Build history of the part. All positions in model axes, mm. A direction names the side the tool comes from. Give positions to 0.01 mm unless a question says otherwise; leave off trailing zeros. Order: outer loops, then holes, each group sorted by start corner. A loop starts at its lowest first (then second) coordinate and runs counter-clockwise, first axis right, second up. Notation, with made-up numbers: (49, 30) - (82, 30) arc R12 ccw to (82, 44) - close; hole circle Ø11 at (12.25, -16.75). An arc over 180 degrees is marked (long way). Use a Markdown table: item, result.
Autodesk Inventor part; units mm, degrees
ref_plane "YZ Plane" through (0, 0, 0) normal (1, 0, 0) x (0, 1, 0)
ref_plane "XZ Plane" through (0, 0, 0) normal (0, 1, 0) x (-1, 0, 0)
ref_plane "XY Plane" through (0, 0, 0) normal (0, 0, 1) x (1, 0, 0)
sketch "Sketch1" plane through (0, 0, 0) normal (0, 0, 1) x (1, 0, 0)
  line L0 (-79.2915, 39.2514) -> (-13.7915, 39.2514)
  line L1 (-13.7915, 39.2514) -> (-13.7915, 1.2514)
  line L2 (-13.7915, 1.2514) -> (-79.2915, 1.2514)
  line L3 (-79.2915, 1.2514) -> (-79.2915, 39.2514)
  point P0 (0, 0)
extrude "Extrusion1" add sketch "Sketch1" along normal blind 1.5
sketch "Sketch2" plane through (0, 0, 1.5) normal (0, 0, 1) x (1, 0, 0)
  line L0 (-13.7915, 39.2514) -> (-13.7915, 1.2514)
  line L1 (-79.2915, 39.2514) -> (-13.7915, 39.2514)
  line L2 (-79.2915, 1.2514) -> (-79.2915, 39.2514)
  line L3 (-13.7915, 1.2514) -> (-79.2915, 1.2514)
  line L4 (-79.2915, 37.2514) -> (-15.7915, 37.2514)
  line L5 (-15.7915, 37.2514) -> (-15.7915, 3.2514)
  line L6 (-15.7915, 3.2514) -> (-79.2915, 3.2514)
  point P0 (0, 0)
  dimension "d2" = 2
  dimension "d3" = 2
  dimension "d4" = 2
extrude "Extrusion2" add sketch "Sketch2" along normal blind 14.5 contours L0 L3 L2 L6 L5 L4 L1
sketch "Sketch3" plane through (-13.7915, 1.2514, 0) normal (1, 0, 0) x (0, 0, -1)
  line L0 (0, 0) -> (-16, 0)
  line L1 (0, 38) -> (0, 0)
  line L2 (0, 38) -> (-16, 38)
  line L3 (-16, 38) -> (-16, 0)
  arc A0 (-13, 24.3) -> (-13, 30.7) centre (-13, 27.5) ccw
  line L4 (-13, 30.7) -> (-16, 30.7)
  line L5 (-13, 24.3) -> (-16, 24.3)
  arc A1 (-13, 7.3) -> (-13, 13.7) centre (-13, 10.5) ccw
  line L6 (-13, 7.3) -> (-16, 7.3)
  line L7 (-13, 13.7) -> (-16, 13.7)
  point P0 (0, -1.2514)
  dimension "d7" = 13
  dimension "d8" = 10.5
  dimension "d9" = 3.2
  dimension "d10" = 13
  dimension "d11" = 10.5
extrude "Extrusion3" cut sketch "Sketch3" against normal blind 13 contours L3 L7 A1 L6 | L4 A0 L5 L3
sketch "Sketch4" plane through (0, 0, 0) normal (0, 0, -1) x (-1, 0, 0)
  line L0 (21.3312, 42.5198) -> (19.2419, 38.901)
  arc A0 (21.3312, 42.5198) -> (21.3312, 44.5198) centre (19.5992, 43.5198) ccw
  line L1 (19.8192, 47.1386) -> (21.3312, 44.5198)
  arc A1 (19.8192, 47.1386) -> (18.0872, 48.1386) centre (18.0872, 46.1386) ccw
  line L2 (15.0633, 48.1386) -> (18.0872, 48.1386)
  arc A2 (15.0633, 48.1386) -> (13.3312, 47.1386) centre (15.0633, 46.1386) ccw
  line L3 (11.8192, 44.5198) -> (13.3312, 47.1386)
  arc A3 (11.8192, 44.5198) -> (11.8192, 42.5198) centre (13.5513, 43.5198) ccw
  line L4 (12.8585, 40.7198) -> (11.8192, 42.5198)
  circle A4 centre (16.5752, 43.5198) radius 1.65
  line L5 (12.8585, 40.7198) -> (13.7938, 39.0998)
  line L6 (13.7938, 39.0998) -> (19.3567, 39.0998)
  point P0 (0, 0)
  point P1 (16.0419, 38.7198)
extrude "Extrusion4" add sketch "Sketch4" against normal blind 16
sketch "Sketch5" plane through (-79.2915, 1.2514, 0) normal (-1, 0, 0) x (0, 0, 1)
  line L0 (1.5, 2) -> (1.5, 36)
  line L1 (0, 38) -> (16, 38)
  line L2 (0, 0) -> (0, 38)
  line L3 (0, 0) -> (16, 0)
  line L4 (1.5, 36) -> (1.5, 38)
  line L5 (1.5, 2) -> (1.5, 0)
  point P0 (0, -1.2514)
extrude "Extrusion5" add sketch "Sketch5" along normal blind 8
sketch "Sketch6" plane through (0, 0, 1.5) normal (0, 0, 1) x (1, 0, 0)
  line L0 (-15.7915, 37.2514) -> (-79.2915, 37.2514)
  line L1 (-79.2915, 3.2514) -> (-15.7915, 3.2514)
  line L2 (-15.7915, 3.2514) -> (-15.7915, 37.2514)
  line L3 (-69.2915, 37.2514) -> (-66.2915, 37.2514)
  line L4 (-66.2915, 37.2514) -> (-66.2915, 3.2514)
  line L5 (-66.2915, 3.2514) -> (-69.2915, 3.2514)
  line L6 (-69.2915, 3.2514) -> (-69.2915, 37.2514)
  line L7 (-40.7915, 37.2514) -> (-37.7915, 37.2514)
  line L8 (-37.7915, 37.2514) -> (-37.7915, 3.2514)
  line L9 (-37.7915, 3.2514) -> (-40.7915, 3.2514)
  line L10 (-40.7915, 3.2514) -> (-40.7915, 37.2514)
  point P0 (0, 0)
  dimension "d18" = 3
  dimension "d19" = 3
  dimension "d20" = 22
  dimension "d21" = 10
extrude "Extrusion6" add sketch "Sketch6" along normal blind 5.2 contours L8 L1 L10 L0 | L4 L1 L6 L0
sketch "Sketch7" plane through (0, 0, 0) normal (0, 0, -1) x (-1, 0, 0)
  line L0 (87.2915, 39.2514) -> (19.4442, 39.2514)
  line L1 (18.0872, 35.2514) -> (20.0872, 35.2514)
  line L2 (20.0872, 35.2514) -> (20.0872, 5.2514)
  line L3 (20.0872, 5.2514) -> (18.0872, 5.2514)
  line L4 (18.0872, 5.2514) -> (18.0872, 35.2514)
  circle A0 centre (19.0872, 35.2514) radius 1
  circle A1 centre (19.0872, 5.2514) radius 1
  point P0 (0, 0)
  dimension "d24" = 2
  dimension "d25" = 30
  dimension "d26" = 4
  dimension "d32" = 2
  dimension "d33" = 2
extrude "Extrusion7" cut sketch "Sketch7" against normal blind 2
pattern_linear "Rectangular Pattern1" count 5 spacing 4 along (-1, 0, 0) of "Extrusion7"
sketch "Sketch8" plane through (0, 0, 0) normal (0, 0, -1) x (-1, 0, 0)
  line L0 (13.7915, 1.2514) -> (87.2915, 1.2514)
  line L1 (87.2915, 1.2514) -> (87.2915, 39.2514)
  line L2 (42.2915, 32.2514) -> (44.2915, 32.2514)
  line L3 (44.2915, 32.2514) -> (44.2915, 8.2514)
  line L4 (44.2915, 8.2514) -> (42.2915, 8.2514)
  line L5 (42.2915, 8.2514) -> (42.2915, 32.2514)
  circle A0 centre (43.2915, 32.2514) radius 1
  circle A1 centre (43.2915, 8.2514) radius 1
  point P0 (0, 0)
  dimension "d34" = 2
  dimension "d35" = 24
  dimension "d36" = 43
  dimension "d37" = 7
extrude "Extrusion8" cut sketch "Sketch8" against normal blind 2
pattern_linear "Rectangular Pattern2" count 2 spacing 4 along (-1, 0, 0) of "Extrusion8"
sketch "Sketch9" plane through (0, 0, 0) normal (0, 0, -1) x (-1, 0, 0)
  line L0 (87.2915, 39.2514) -> (19.4442, 39.2514)
  line L1 (55.3139, 35.2514) -> (57.3139, 35.2514)
  line L2 (57.3139, 35.2514) -> (57.3139, 5.2514)
  line L3 (57.3139, 5.2514) -> (55.3139, 5.2514)
  line L4 (55.3139, 5.2514) -> (55.3139, 35.2514)
  circle A0 centre (56.3139, 35.2514) radius 1
  circle A1 centre (56.3139, 5.2514) radius 1
  point P0 (0, 0)
  dimension "d43" = 30
  dimension "d44" = 4
extrude "Extrusion9" cut sketch "Sketch9" against normal blind 2
pattern_linear "Rectangular Pattern3" count 3 spacing 4 along (-1, 0, 0) of "Extrusion9"
sketch "Sketch11" plane through (0, 0, 0) normal (0, 0, -1) x (-1, 0, 0)
  line L0 (87.2915, 1.2514) -> (87.2915, 39.2514)
  line L1 (87.2915, 39.2514) -> (19.4442, 39.2514)
  circle A0 centre (84.7915, 32.3514) radius 1.5
  circle A1 centre (84.7915, 8.1514) radius 1.5
  point P0 (0, 0)
  dimension "d50" = 2.5
  dimension "d51" = 2.5
  dimension "d52" = 24.2
  dimension "d53" = 6.9
extrude "Extrusion10" cut sketch "Sketch11" against normal blind 10
chamfer "Chamfer1" distance 0.5 angle 45 13 edges at (-50.5415, 1.2514, 0) (-13.7915, 20.1776, 0) (-13.7915, 1.2514, 8) (-53.3678, 39.2514, 0) (-20.3877, 40.8856, 0) (-21.5992, 43.5198, 0) (-20.5752, 45.8292, 0) (-19.0872, 47.8707, 0) (-16.5752, 48.1386, 0) (-14.0633, 47.8707, 0) (-12.5752, 45.8292, 0) (-11.5513, 43.5198, 0) (-12.8054, 40.8118, 0)
sketch "Sketch12" plane through (0, 0, 0) normal (0, 0, -1) x (-1, 0, 0)
  line L0 (87.2915, 1.7514) -> (87.2915, 38.7514)
  circle A0 centre (84.7915, 32.3514) radius 1.5
  circle A1 centre (84.7915, 8.1514) radius 1.5
  line L1 (87.2915, 39.2514) -> (79.2915, 39.2514)
  line L2 (79.2915, 39.2514) -> (79.2915, 1.2514)
  line L3 (79.2915, 1.2514) -> (87.2915, 1.2514)
  line L4 (87.2915, 1.2514) -> (87.2915, 39.2514)
  line L5 (14.2915, 1.2514) -> (87.2915, 1.2514)
  point P0 (0, 0)
  dimension "d59" = 38
  dimension "d60" = 8
  dimension "d61" = 0
  dimension "d64" = 0
extrude "Extrusion11" add sketch "Sketch12" against normal blind 1
sketch "Sketch13" plane through (0, 0, 0) normal (0, 0, -1) x (-1, 0, 0)
  circle A0 centre (16.5752, 43.5198) radius 1.65
  circle A1 centre (16.5752, 43.5198) radius 3.5
  point P0 (0, 0)
extrude "Extrusion12" cut sketch "Sketch13" against normal blind 3
properties part number "case add on sdr botom"
1) Two-plate mould, pull along Y, no slides. Class faces 1 (the flat face through (-35, 38, 16)), 2 (the cylindrical face through (-19.1, 47.863, 8.142)), 3 (the flat face through (-66.292, 20, 4)): +Y half, -Y half, draft (parallel to the pull), parting line (faces both ways), or undercut.
Computed:
| item | result |
|---|---|
| face 1 | draft |
| face 2 | +Y half |
| face 3 | undercut |
2) Tool access for faces 4 (the flat face through (-29, 20, 1.5)), 5 (the flat face through (-79.292, 38, 9)), 6 (the flat face through (-39, 20, 6.7)), 7 (the cylindrical face through (-27.07, 4.25, 0.74)): list every direction of +Z, -Z, +X, -X, +Y, -Y with a clear straight run to the whole face (end or side of a thin tool).
Computed:
| item | result |
|---|---|
| face 4 | +Z |
| face 5 | +Z, -X, +Y, -Y |
| face 6 | +Z, -X |
| face 7 | +Z, -Z |
3) Wall check: line 1 (X direction, y = 32.5, z = 1.75); line 2 (Y direction, x = -60.5, z = 6.25); line 3 (X direction, y = 36, z = 12.75). Give the ranges that are in metal, low to high. Write a range as from..to.
Computed:
| item | result |
|---|---|
| line 1 | x = -69.29..-66.29, -40.79..-37.79, -15.79..-13.79 |
| line 2 | y = 1.25..3.25, 37.25..39.25 |
| line 3 | x = -15.79..-13.79 |
4) Slice it at D-D (y = 30). State how many separate pieces and enclosed holes the cut face has, and give its area (3 significant figures).
Computed:
| item | result |
|---|---|
| separate pieces | 11 |
| enclosed holes | 0 |
| area | 128 mm² |
5) Slice it at C-C (z = 4.75). Write the cut outline in (x, y).
Computed:
| item | result |
|---|---|
| outline | (-79.29, 1.25) - (-14.29, 1.25) - (-13.79, 1.75) - (-13.79, 39.1) - (-12.86, 40.72) - (-11.82, 42.52) arc R2 ccw to (-11.82, 44.52) - (-13.33, 47.14) arc R2 ccw to (-15.06, 48.14) - (-18.09, 48.14) arc R2 ccw to (-19.82, 47.14) - (-21.33, 44.52) arc R2 ccw to (-21.33, 42.52) - (-19.44, 39.25) - (-79.29, 39.25) - (-79.29, 37.25) - (-69.29, 37.25) - (-69.29, 3.25) - (-79.29, 3.25) - close; hole (-66.29, 3.25) - (-40.79, 3.25) - (-40.79, 37.25) - (-66.29, 37.25) - close; hole (-37.79, 3.25) - (-15.79, 3.25) - (-15.79, 37.25) - (-37.79, 37.25) - close; hole circle Ø3.3 at (-16.58, 43.52) |
6) Slice it at B-B (y = 38). Write the cut outline in (x, z).
Computed:
| item | result |
|---|---|
| outline | (-87.29, 0) - (-14.29, 0) - (-13.79, 0.5) - (-13.79, 16) - (-79.29, 16) - (-79.29, 1.5) - (-87.29, 1.5) - close |
7) Pin check, flat tips, straight feed: P1, Ø3.5, axis at x = -67.5, y = 17, coming from the +Z side; P2, Ø4, axis at x = -84.79, y = 8.15, coming from the +Z side; P3, Ø0.6, axis at y = 1.5, z = 0.5, coming from the +X side. Stop position of each tip, or through.
Computed:
| item | result |
|---|---|
| P1 | stops at z = 6.7 |
| P2 | stops at z = 1.5 |
| P3 | stops at x = -13.79 |
8) Slice it at A-A (z = 15). Write the cut outline in (x, y).
Computed:
| item | result |
|---|---|
| outline | (-79.29, 1.25) - (-14.29, 1.25) - (-13.79, 1.75) - (-13.79, 8.55) - (-15.79, 8.55) - (-15.79, 3.25) - (-79.29, 3.25) - close; (-79.29, 37.25) - (-15.79, 37.25) - (-15.79, 31.95) - (-13.79, 31.95) - (-13.79, 39.1) - (-12.86, 40.72) - (-11.82, 42.52) arc R2 ccw to (-11.82, 44.52) - (-13.33, 47.14) arc R2 ccw to (-15.06, 48.14) - (-18.09, 48.14) arc R2 ccw to (-19.82, 47.14) - (-21.33, 44.52) arc R2 ccw to (-21.33, 42.52) - (-19.44, 39.25) - (-79.29, 39.25) - close; (-15.79, 14.95) - (-13.79, 14.95) - (-13.79, 25.55) - (-15.79, 25.55) - close; hole circle Ø3.3 at (-16.58, 43.52) |
